Build history of the part. All positions in model axes, mm. Face numbers are marked on the shaded views. Give positions to 0.01 mm unless a question says otherwise; leave off trailing zeros. Order: outer loops, then holes, each group sorted by start corner. A loop starts at its lowest first (then second) coordinate and runs counter-clockwise, first axis right, second up. Notation, with made-up numbers: M 21,-37.75 L 57,-37.75 A13 ccw 57,-18.75 Z; hole C 31,-38 d2. An arc over 180 degrees is marked long. Use CSV: the item, a comma, the result in double quotes. Start each with the question number.
Item 1: Band-saw the part on C-C on y = 22.5. Write the cut outline in (x, z).
Item 2: Band-saw the part on A-A on x = 2.25. Write the cut outline in (y, z), plus the area to 3 significant figures.
Item 3: Pin check, flat tips, straight feed: P1, Ø2, axis at x = 2, z = -0.5, coming from the +Y side; P2, Ø8, axis at y = 18.5, z = -4, coming from the -X side; P3, Ø3, axis at x = 0.5, y = -3.5, coming from the -Z side. Stop position of each tip, or through.
Item 4: Wall check: line 1 along Z through (x, y) = (3.8, 41.5); line 2 along Y through (x, z) = (2.8, -1); line 3 along X through (y, z) = (31, 10). Give the ranges that are in metal, low to high.
Item 5: Two-plate mould, pull along Z, no slides. Class the marked faces 1 and 2: pulls with the +Z half, pulls with the -Z half, needs draft (parallel to the pull), parting line crosses it, or undercut.
Item 6: Band-saw the part on B-B on z = 4.5. Write the cut outline in (x, y).
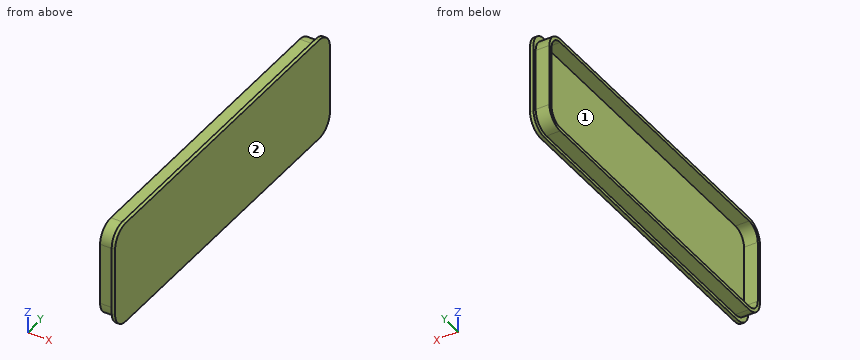
from build123d import *

# Parameters (mm, degrees)
F1_DEPTH = 5
F3_DEPTH = 4
F4_T     = -1


with BuildPart() as f1:
    # F0 (on Right) → F1 (new body)
    with BuildSketch(Plane.YZ):
        with BuildLine():
            ThreePointArc((-50, -10), (-48.5355339059, -13.5355339059), (-45, -15))
            Line((-45, -15), (45, -15))
            ThreePointArc((45, -15), (48.5355339059, -13.5355339059), (50, -10))
            Line((50, -10), (50, 10))
            ThreePointArc((50, 10), (48.5355339059, 13.5355339059), (45, 15))
            Line((45, 15), (-45, 15))
            ThreePointArc((-45, 15), (-48.5355339059, 13.5355339059), (-50, 10))
            Line((-50, 10), (-50, -10))
        make_face()
    extrude(amount=F1_DEPTH)

    # F2 (on face) → F3 (cut)
    with BuildSketch(Plane(origin=(0, 0, 0), x_dir=(0, -1, 0), z_dir=(-1, 0, 0))):
        with BuildLine():
            Line((-45, -15), (45, -15))
            ThreePointArc((45, -15), (48.5355339059, -13.5355339059), (50, -10))
            Line((50, -10), (50, 10))
            ThreePointArc((50, 10), (48.5355339059, 13.5355339059), (45, 15))
            Line((45, 15), (-45, 15))
            ThreePointArc((-45, 15), (-48.5355339059, 13.5355339059), (-50, 10))
            Line((-50, 10), (-50, -10))
            ThreePointArc((-50, -10), (-48.5355339059, -13.5355339059), (-45, -15))
        make_face()
        with BuildLine():
            ThreePointArc((49, -9), (47.5355339059, -12.5355339059), (44, -14))
            Line((44, -14), (-44, -14))
            ThreePointArc((-44, -14), (-47.5355339059, -12.5355339059), (-49, -9))
            Line((-49, -9), (-49, 9))
            ThreePointArc((-49, 9), (-47.5355339059, 12.5355339059), (-44, 14))
            Line((-44, 14), (44, 14))
            ThreePointArc((44, 14), (47.5355339059, 12.5355339059), (49, 9))
            Line((49, 9), (49, -9))
        make_face(mode=Mode.SUBTRACT)
    extrude(amount=-F3_DEPTH, mode=Mode.SUBTRACT)

    # F4
    f4_openings = [f1.faces().sort_by_distance(p)[0] for p in [
        (0, 0, 0),
    ]]
    offset(amount=F4_T, openings=f4_openings, kind=Kind.INTERSECTION)


solid = f1.part
Model answer:
1,outline,"M 0,-14 L 4,-14 L 4,-15 L 5,-15 L 5,15 L 4,15 L 4,14 L 0,14 L 0,13 L 4,13 L 4,-13 L 0,-13 Z"
2,outline,"M -49,-9 A5 ccw -44,-14 L 44,-14 A5 ccw 49,-9 L 49,9 A5 ccw 44,14 L -44,14 A5 ccw -49,9 Z; hole M -48,-9 A4 ccw -44,-13 L 44,-13 A4 ccw 48,-9 L 48,9 A4 ccw 44,13 L -44,13 A4 ccw -48,9 Z"
2,area,"240 mm^2"
3,P1,"stops at y = 49"
3,P2,"stops at x = 4"
3,P3,"stops at z = -14"
4,line 1,"z = -14 to -13, 13 to 14"
4,line 2,"y = -49 to -48, 48 to 49"
4,line 3,"x = 4 to 5"
5,face 1,"undercut"
5,face 2,"needs draft"
6,outline,"M 0,-49 L 4,-49 L 4,-50 L 5,-50 L 5,50 L 4,50 L 4,49 L 0,49 L 0,48 L 4,48 L 4,-48 L 0,-48 Z"
